```python
from build123d import *

# Parameters (mm, degrees)
SKETCH1_W           = 160
SKETCH1_H           = 220
BOSS_EXTRUDE1_DEPTH = 3
SKETCH3_R           = 1.5
CUT_EXTRUDE1_DEPTH  = 3
SKETCH4_R           = 1.5
CUT_EXTRUDE2_DEPTH  = 3
SKETCH5_R           = 1.5
CUT_EXTRUDE3_DEPTH  = 3
SKETCH6_R           = 0.635
CUT_EXTRUDE4_DEPTH  = 3
SKETCH7_W           = 30
SKETCH7_H           = 18.607589123
CUT_EXTRUDE5_DEPTH  = 3
SKETCH8_W           = 22
SKETCH8_H           = 179.95337022
CUT_EXTRUDE6_DEPTH  = 3
SKETCH10_R          = 2
CUT_EXTRUDE7_DEPTH  = 3
CUT_EXTRUDE8_DEPTH  = 3
FILLET1_R           = 10
FILLET2_R           = 10
FILLET3_R           = 10
CUT_EXTRUDE9_DEPTH  = 10
SKETCH13_R          = 16
CUT_EXTRUDE10_DEPTH = 10
CUT_EXTRUDE11_DEPTH = 2


with BuildPart() as part:
    # Sketch1 → Boss-Extrude1 (new body)
    with BuildSketch(Plane(origin=(0, 0, 0), x_dir=(1, 0, 0), z_dir=(0, 1, 0))):
        Rectangle(SKETCH1_W, SKETCH1_H)
    extrude(amount=BOSS_EXTRUDE1_DEPTH)

    # Sketch3 → Cut-Extrude1 (cut)
    with BuildSketch(Plane(origin=(0, 3, 0), x_dir=(1, 0, 0), z_dir=(0, 1, 0))):
        with Locations(Location((-59.03, 88.2, 0), (0, 0, 270))):
            Circle(SKETCH3_R)
        with Locations(Location((-72.63, 88.2, 0), (0, 0, 270))):
            Circle(SKETCH3_R)
        with Locations(Location((-59.03, 103.8, 0), (0, 0, 270))):
            Circle(SKETCH3_R)
        with Locations(Location((-72.63, 103.8, 0), (0, 0, 270))):
            Circle(SKETCH3_R)
        with Locations(Location((72.63, 103.8, 0), (0, 0, 90))):
            Circle(SKETCH3_R)
        with Locations(Location((59.03, 103.8, 0), (0, 0, 90))):
            Circle(SKETCH3_R)
        with Locations(Location((72.63, 88.2, 0), (0, 0, 90))):
            Circle(SKETCH3_R)
        with Locations(Location((59.03, 88.2, 0), (0, 0, 90))):
            Circle(SKETCH3_R)
    extrude(amount=-CUT_EXTRUDE1_DEPTH, mode=Mode.SUBTRACT)

    # Sketch4 → Cut-Extrude2 (cut)
    with BuildSketch(Plane(origin=(0, 3, 0), x_dir=(1, 0, 0), z_dir=(0, 1, 0))):
        with Locations(Location((-19.65, 100.584248084, 0), (0, 0, 270))):
            Circle(SKETCH4_R)
        with Locations(Location((19.65, 100.584248084, 0), (0, 0, 90))):
            Circle(SKETCH4_R)
        with Locations(Location((19.65, 61.284248084, 0), (0, 0, 270))):
            Circle(SKETCH4_R)
        with Locations(Location((-19.65, 61.284248084, 0), (0, 0, 90))):
            Circle(SKETCH4_R)
    extrude(amount=-CUT_EXTRUDE2_DEPTH, mode=Mode.SUBTRACT)

    # Sketch5 → Cut-Extrude3 (cut)
    with BuildSketch(Plane(origin=(0, 3, 0), x_dir=(1, 0, 0), z_dir=(0, 1, 0))):
        with Locations(Location((0, 20, 0), (0, 0, 270))):
            Circle(SKETCH5_R)
        with Locations(Location((0, -20, 0), (0, 0, 270))):
            Circle(SKETCH5_R)
    extrude(amount=-CUT_EXTRUDE3_DEPTH, mode=Mode.SUBTRACT)

    # Sketch6 → Cut-Extrude4 (cut)
    with BuildSketch(Plane(origin=(0, 3, 0), x_dir=(1, 0, 0), z_dir=(0, 1, 0))):
        with Locations(Location((-20.83, 48.244137144, 0), (0, 0, 270))):
            Circle(SKETCH6_R)
        with Locations(Location((20.83, 48.244137144, 0), (0, 0, 90))):
            Circle(SKETCH6_R)
        with Locations(Location((20.83, 31.984137144, 0), (0, 0, 270))):
            Circle(SKETCH6_R)
        with Locations(Location((-20.83, 31.984137144, 0), (0, 0, 90))):
            Circle(SKETCH6_R)
    extrude(amount=-CUT_EXTRUDE4_DEPTH, mode=Mode.SUBTRACT)

    # Sketch7 → Cut-Extrude5 (cut)
    with BuildSketch(Plane(origin=(0, 3, 0), x_dir=(1, 0, 0), z_dir=(0, 1, 0))):
        with BuildLine():
            Line((-42, -91), (-25, -91))
            ThreePointArc((-25, -91), (-23.5, -92.5), (-25, -94))
            Line((-25, -94), (-42, -94))
            ThreePointArc((-42, -94), (-43.5, -92.5), (-42, -91))
        make_face()
        with Locations((0, -85.183731289)):
            Rectangle(SKETCH7_W, SKETCH7_H)
        with BuildLine():
            Line((42, -91), (25, -91))
            ThreePointArc((25, -91), (23.5, -92.5), (25, -94))
            Line((25, -94), (42, -94))
            ThreePointArc((42, -94), (43.5, -92.5), (42, -91))
        make_face()
    extrude(amount=-CUT_EXTRUDE5_DEPTH, mode=Mode.SUBTRACT)

    # Sketch8 → Cut-Extrude6 (cut)
    with BuildSketch(Plane(origin=(0, 3, 0), x_dir=(1, 0, 0), z_dir=(0, 1, 0))):
        with Locations((69, -20.02331489)):
            Rectangle(SKETCH8_W, SKETCH8_H)
        with Locations((-69, -20.02331489)):
            Rectangle(SKETCH8_W, SKETCH8_H)
    extrude(amount=-CUT_EXTRUDE6_DEPTH, mode=Mode.SUBTRACT)

    # Sketch10 → Cut-Extrude7 (cut)
    with BuildSketch(Plane(origin=(0, 3, 0), x_dir=(1, 0, 0), z_dir=(0, 1, 0))):
        with Locations(Location((-20, -51.206202612, 0), (0, 0, 270))):
            Circle(SKETCH10_R)
        with Locations(Location((20, -51.206202612, 0), (0, 0, 270))):
            Circle(SKETCH10_R)
    extrude(amount=-CUT_EXTRUDE7_DEPTH, mode=Mode.SUBTRACT)

    # Sketch11 → Cut-Extrude8 (cut)
    with BuildSketch(Plane(origin=(0, 3, 0), x_dir=(1, 0, 0), z_dir=(0, 1, 0))):
        Polygon((-80, 79.063576574), (-38.06764798, 79.063576574), (-38.06764798, -80.039670112), (-51.407592999, -80.039670112), (-51.407592999, -110), (-58, -110), (-58, 69.95337022), (-80, 69.95337022), align=None)
        Polygon((80, 69.95337022), (80, 79.063576574), (38.06764798, 79.063576574), (38.06764798, -80.039670112), (51.407592999, -80.039670112), (51.407592999, -110), (58, -110), (58, 69.95337022), align=None)
    extrude(amount=-CUT_EXTRUDE8_DEPTH, mode=Mode.SUBTRACT)

    # Fillet1
    fillet1_edges = [part.edges().sort_by_distance(p)[0] for p in [
        (-51.407592999, 1.5, 110),
    ]]
    fillet(fillet1_edges, radius=FILLET1_R)

    # Fillet2
    fillet2_edges = [part.edges().sort_by_distance(p)[0] for p in [
        (-80, 1.5, -79.063576574),
        (-51.407592999, 1.5, 80.039670112),
        (80, 1.5, -79.063576574),
        (-80, 1.5, -110),
        (80, 1.5, -110),
    ]]
    fillet(fillet2_edges, radius=FILLET2_R)

    # Fillet3
    fillet3_edges = [part.edges().sort_by_distance(p)[0] for p in [
        (51.407592999, 1.5, 110),
        (51.407592999, 1.5, 80.039670112),
    ]]
    fillet(fillet3_edges, radius=FILLET3_R)

    # Sketch12 → Cut-Extrude9 (cut)
    with BuildSketch(Plane(origin=(0, 3, 0), x_dir=(1, 0, 0), z_dir=(0, 1, 0))):
        with BuildLine():
            Line((-36.56764798, 36.063576574), (-36.56764798, 76.063576574))
            ThreePointArc((-36.56764798, 76.063576574), (-35.06764798, 77.563576574), (-33.56764798, 76.063576574))
            Line((-33.56764798, 76.063576574), (-33.56764798, 36.063576574))
            ThreePointArc((-33.56764798, 36.063576574), (-35.06764798, 34.563576574), (-36.56764798, 36.063576574))
        make_face()
        with BuildLine():
            Line((36.56764798, 36.063576574), (36.56764798, 76.063576574))
            ThreePointArc((36.56764798, 76.063576574), (35.06764798, 77.563576574), (33.56764798, 76.063576574))
            Line((33.56764798, 76.063576574), (33.56764798, 36.063576574))
            ThreePointArc((33.56764798, 36.063576574), (35.06764798, 34.563576574), (36.56764798, 36.063576574))
        make_face()
    extrude(amount=-CUT_EXTRUDE9_DEPTH, mode=Mode.SUBTRACT)

    # Sketch13 → Cut-Extrude10 (cut)
    with BuildSketch(Plane(origin=(0, 3, 0), x_dir=(1, 0, 0), z_dir=(0, 1, 0))):
        with Locations(Location((0, -51.206202612, 0), (0, 0, 270))):
            Circle(SKETCH13_R)
    extrude(amount=-CUT_EXTRUDE10_DEPTH, mode=Mode.SUBTRACT)

    # Sketch14 → Cut-Extrude11 (cut)
    with BuildSketch(Plane(origin=(0, 3, 0), x_dir=(1, 0, 0), z_dir=(0, 1, 0))):
        with BuildLine():
            Line((-36.56764798, -73.039670112), (-36.56764798, -33.039670112))
            ThreePointArc((-36.56764798, -33.039670112), (-35.06764798, -31.539670112), (-33.56764798, -33.039670112))
            Line((-33.56764798, -33.039670112), (-33.56764798, -73.039670112))
            ThreePointArc((-33.56764798, -73.039670112), (-35.06764798, -74.539670112), (-36.56764798, -73.039670112))
        make_face()
        with BuildLine():
            Line((36.56764798, -73.039670112), (36.56764798, -33.039670112))
            ThreePointArc((36.56764798, -33.039670112), (35.06764798, -31.539670112), (33.56764798, -33.039670112))
            Line((33.56764798, -33.039670112), (33.56764798, -73.039670112))
            ThreePointArc((33.56764798, -73.039670112), (35.06764798, -74.539670112), (36.56764798, -73.039670112))
        make_face()
    extrude(amount=-CUT_EXTRUDE11_DEPTH, mode=Mode.SUBTRACT)


solid = part.part
```
Model file for the job. Use its own axes, mm. A direction names the side the tool comes from. Coordinates: 2 decimals unless noted, no trailing zeros. Order: outer loops, then holes, each group sorted by start corner. A loop starts at its lowest first (then second) coordinate and runs counter-clockwise, first axis right, second up. Notation, with made-up numbers: (54.25, -6) - (80.25, -6) arc R18 ccw to (80.25, 6) - close; hole circle Ø4 at (65.25, 19.25). An arc over 180 degrees is marked (long way). Return JSON: item names as keys, results as strings. Group by question number.
1) Probe line 1 (X direction, y = 0.9, z = -39); line 2 (Z direction, x = 59.03, y = 0.85); line 3 (X direction, y = 2.1, z = -103.8). List the from-to ranges inside material, lowest first. Write a range as from..to.
2) Saw through at A-A, the plane z = -55. Write the cut outline in (x, y), plus the area to 3 significant figures.
3) Saw through at B-B, the plane y = 1.9. Count the separate pieces of the cut face and the enclosed holes in it, plus the area to 3 significant figures.
4) Mould opens along Z. For faces 3 (the cylindrical face through (-48.56, 1.48, 83.05)), 4 (the cylindrical face through (-48.4, 1.48, 107.15)), 5 (the cylindrical face through (-77.15, 1.52, -106.99)) say: released by +Z, released by -Z, zero draft, split by the parting line, or undercut.
5) Saw through at C-C, the plane x = 54.5. Write the cut outline in (y, z), plus the area to 3 significant figures.
6) Flat gauge pins, fed straight in: P1, Ø2.5, axis at x = -19.65, z = -61.28, coming from the -Y side; P2, Ø1, axis at y = 0.5, z = -18.5, coming from the +X side; P3, Ø6.5, axis at x = 20, z = 51.21, coming from the +Y side; P4, Ø0.9, axis at y = 1.5, z = -48.5, coming from the -X side. Where does each tip first touch, or does it go through?
7) Tool access for faces 1 (the cylindrical face through (48.56, 1.48, 83.05)), 2 (the cylindrical face through (76.993, 1.479, -81.915)): list every direction of +Z, -Z, +X, -X, +Y, -Y with a clear straight run to the whole face (end or side of a thin tool).
Values found:
{
 "1": {"line 1": "x = -38.07..-36.57, -33.57..33.57, 36.57..38.07", "line 2": "z = -110..-105.3, -102.3..-89.7, -86.7..-79.06", "line 3": "x = -79.25..-74.13, -71.13..-60.53, -57.53..57.53, 60.53..71.13, 74.13..79.25"},
 "2": {"outline": "(-38.07, 0) - (-36.57, 0) - (-36.57, 3) - (-38.07, 3) - close; (-33.57, 0) - (33.57, 0) - (33.57, 3) - (-33.57, 3) - close; (36.57, 0) - (38.07, 0) - (38.07, 3) - (36.57, 3) - close", "area": "210 mm²"},
 "3": {"separate pieces": "1", "enclosed holes": "28", "area": "17,900 mm²"},
 "4": {"face 3": "undercut", "face 4": "released by +Z", "face 5": "released by -Z"},
 "5": {"outline": "(0, -110) - (3, -110) - (3, -79.06) - (0, -79.06) - close", "area": "92.8 mm²"},
 "6": {"P1": "passes through", "P2": "stops at x = 38.07", "P3": "stops at y = 3", "P4": "stops at x = -38.07"},
 "7": {"face 1": "+X, +Y, -Y", "face 2": "+Z, +X, +Y, -Y"}
}
